```python
from build123d import *

# Parameters (mm, degrees)
SALIENTE_EXTRUIR1_DEPTH = 6
CROQUIS7_R              = 40
SALIENTE_EXTRUIR5_DEPTH = 6
SALIENTE_EXTRUIR3_DEPTH = 6
CROQUIS6_R              = 1.75
SALIENTE_EXTRUIR4_DEPTH = 6
CROQUIS8_W              = 6
CROQUIS8_H              = 6
CORTAR_EXTRUIR1_DEPTH   = 25
CROQUIS9_R              = 40
CORTAR_EXTRUIR2_DEPTH   = 18


with BuildPart() as part:
    # Croquis1 → Saliente-Extruir1 (new body)
    with BuildSketch(Plane(origin=(0, 0, 0), x_dir=(1, 0, 0), z_dir=(0, 1, 0))):
        with BuildLine():
            Line((-161, 103.5), (-38.791887254, 9.756509788))
            ThreePointArc((-38.791887254, 9.756509788), (-40, 0), (-38.791887254, -9.756509788))
            Line((-38.791887254, -9.756509788), (-161, -103.5))
            Line((-161, -103.5), (-161, -123.5))
            Line((-161, -123.5), (-141, -123.5))
            Line((-141, -123.5), (-22.823766962, -32.84928708))
            ThreePointArc((-22.823766962, -32.84928708), (0, -40), (22.823766962, -32.84928708))
            Line((22.823766962, -32.84928708), (141, -123.5))
            Line((141, -123.5), (161, -123.5))
            Line((161, -123.5), (161, -103.5))
            Line((161, -103.5), (38.791887254, -9.756509788))
            ThreePointArc((38.791887254, -9.756509788), (40, 0), (38.791887254, 9.756509788))
            Line((38.791887254, 9.756509788), (161, 103.5))
            Line((161, 103.5), (161, 123.5))
            Line((161, 123.5), (141, 123.5))
            Line((141, 123.5), (22.823766962, 32.84928708))
            ThreePointArc((22.823766962, 32.84928708), (0, 40), (-22.823766962, 32.84928708))
            Line((-22.823766962, 32.84928708), (-141, 123.5))
            Line((-141, 123.5), (-161, 123.5))
            Line((-161, 123.5), (-161, 103.5))
        make_face()
    extrude(amount=SALIENTE_EXTRUIR1_DEPTH)

    # Croquis7 → Saliente-Extruir5 (add)
    with BuildSketch(Plane(origin=(0, 0, 0), x_dir=(-1, 0, 0), z_dir=(0, -1, 0))):
        Circle(CROQUIS7_R)
    extrude(amount=SALIENTE_EXTRUIR5_DEPTH)

    # Croquis5 → Saliente-Extruir3 (add)
    with BuildSketch(Plane.XZ.offset(6)):
        with BuildLine():
            Line((18.896097481, -21), (-18.896097481, -21))
            ThreePointArc((-18.896097481, -21), (-28.25, 0), (-18.896097481, 21))
            Line((-18.896097481, 21), (-13.25, 21))
            Line((-13.25, 21), (-13.25, -11))
            Line((-13.25, -11), (13.25, -11))
            Line((13.25, -11), (13.25, 21))
            Line((13.25, 21), (18.896097481, 21))
            ThreePointArc((18.896097481, 21), (28.25, 0), (18.896097481, -21))
        make_face()
    extrude(amount=SALIENTE_EXTRUIR3_DEPTH)

    # Croquis6 → Saliente-Extruir4 (add)
    with BuildSketch(Plane.XZ.offset(12)):
        with BuildLine():
            Line((-18.896097481, 21), (-13.25, 21))
            Line((-13.25, 21), (-13.25, 3.5))
            ThreePointArc((-13.25, 3.5), (-13.103553391, 3.146446609), (-12.75, 3))
            Line((-12.75, 3), (12.75, 3))
            ThreePointArc((12.75, 3), (13.103553391, 3.146446609), (13.25, 3.5))
            Line((13.25, 3.5), (13.25, 21))
            Line((13.25, 21), (18.896097481, 21))
            ThreePointArc((18.896097481, 21), (28.25, 0), (18.896097481, -21))
            Line((18.896097481, -21), (-18.896097481, -21))
            ThreePointArc((-18.896097481, -21), (-28.25, 0), (-18.896097481, 21))
        make_face()
        with Locations((-8, -5.75)):
            Circle(CROQUIS6_R, mode=Mode.SUBTRACT)
        with Locations((8, -5.75)):
            Circle(CROQUIS6_R, mode=Mode.SUBTRACT)
    extrude(amount=SALIENTE_EXTRUIR4_DEPTH)

    # Croquis8 → Cortar-Extruir1 (cut, through all)
    with BuildSketch(Plane.XZ.offset(18)):
        with Locations((-20, 0)):
            Rectangle(CROQUIS8_W, CROQUIS8_H)
        with Locations((20, 0)):
            Rectangle(CROQUIS8_W, CROQUIS8_H)
    extrude(amount=-CORTAR_EXTRUIR1_DEPTH, mode=Mode.SUBTRACT)

    # Croquis9 → Cortar-Extruir2 (cut)
    with BuildSketch(Plane(origin=(0, -18, 0), x_dir=(-1, 0, 0), z_dir=(0, -1, 0))):
        Circle(CROQUIS9_R)
    extrude(amount=-CORTAR_EXTRUIR2_DEPTH, mode=Mode.SUBTRACT)


solid = part.part
```
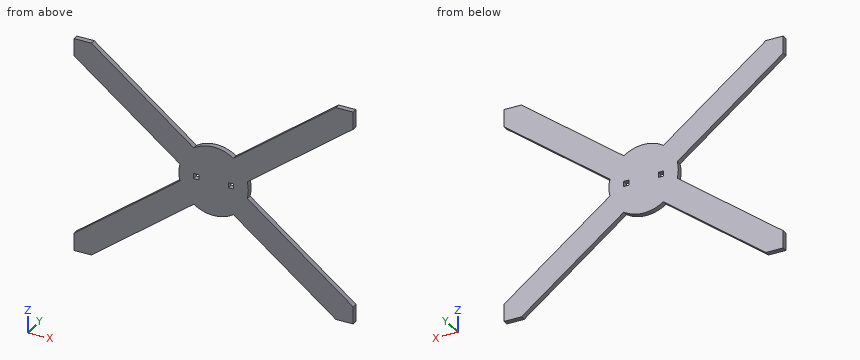
Check sheet for the modelled part. Datum: model origin and axes. Units: mm. Round coordinates to 2 decimals unless told otherwise and drop trailing zeros. Write each loop counter-clockwise with the first axis right and the second up, starting at its lowest first coordinate (ties: lowest second). Pieces come first, ordered by that corner, then holes. Notation, with made-up numbers: (86, 16) -> (116, 16) arc R9 ccw to (116, 20) -> close; hole circle Ø7 at (-24, -9). An arc over 180 degrees is marked (long way). Put each result on its own line as item: value.
(1) Sectioned sample at B-B (x = 112.5). Enter the section's corners in (y, z), plus the area to 3 significant figures.
Values found:
outline: (0, -101.64) -> (6, -101.64) -> (6, -66.3) -> (0, -66.3) -> close; (0, 66.3) -> (6, 66.3) -> (6, 101.64) -> (0, 101.64) -> close
area: 424 mm^2
(2) Sectioned sample at C-C (z = -55). Enter the section's corners in (x, y), plus the area to 3 significant figures.
Values found:
outline: (-97.77, 0) -> (-51.7, 0) -> (-51.7, 6) -> (-97.77, 6) -> close; (51.7, 0) -> (97.77, 0) -> (97.77, 6) -> (51.7, 6) -> close
area: 553 mm^2
(3) Go/stop test with flat-tipped pins: pin 1 Ø3 at (x, y) = (20.5, 2) entering from +Z; pin 2 Ø1.8 at (y, z) = (2, 0.5) entering from -X; pin 3 Ø1.8 at (x, y) = (20, 4) entering from -Z. Record where each tip stops, or that it passes through.
Values found:
pin 1: stops at z = 35.2
pin 2: stops at x = -40
pin 3: stops at z = -35.15
(4) Sectioned sample at A-A (y = 2.8). Enter the section's corners in (x, z).
Values found:
outline: (-161, -123.5) -> (-141, -123.5) -> (-22.82, -32.85) arc R40 ccw to (22.82, -32.85) -> (141, -123.5) -> (161, -123.5) -> (161, -103.5) -> (38.79, -9.76) arc R40 ccw to (38.79, 9.76) -> (161, 103.5) -> (161, 123.5) -> (141, 123.5) -> (22.82, 32.85) arc R40 ccw to (-22.82, 32.85) -> (-141, 123.5) -> (-161, 123.5) -> (-161, 103.5) -> (-38.79, 9.76) arc R40 ccw to (-38.79, -9.76) -> (-161, -103.5) -> close; hole (-23, -3) -> (-17, -3) -> (-17, 3) -> (-23, 3) -> close; hole (17, -3) -> (23, -3) -> (23, 3) -> (17, 3) -> close
(5) Sectioned sample at D-D (z = 18). Enter the section's corners in (x, y), plus the area to 3 significant figures.
Values found:
outline: (-49.54, 0) -> (49.54, 0) -> (49.54, 6) -> (-49.54, 6) -> close
area: 594 mm^2
(6) Material ranges on line 1 (X direction, y = 1.75, z = 0); line 2 (X direction, y = 2.7, z = 33); line 3 (Z direction, x = -94, y = 1.05), recorded low to high.
Values found:
line 1: x = -40 to -23, -17 to 17, 23 to 40
line 2: x = -69.09 to -23.02, -22.61 to 22.61, 23.02 to 69.09
line 3: z = -87.45 to -52.11, 52.11 to 87.45
